The listing builds one solid part. Answer for the finished solid, in the listing's coordinates (mm). Face numbers are marked on the shaded views. A direction names the side the tool comes from. Give positions to 0.01 mm unless a question says otherwise; leave off trailing zeros. Write each loop counter-clockwise with the first axis right and the second up, starting at its lowest first coordinate (ties: lowest second). Pieces come first, ordered by that corner, then holes.
```python
from build123d import *

# Parameters (mm, degrees)
BOSS_EXTRUDE2_DEPTH = 10
FILLET3_R           = 28
SKETCH4_W           = 22
SKETCH4_H           = 48
BOSS_EXTRUDE4_DEPTH = 20
SKETCH9_W           = 18
SKETCH9_H           = 48
BOSS_EXTRUDE6_DEPTH = 60
CUT_EXTRUDE2_DEPTH  = 60
SKETCH12_W          = 18
SKETCH12_H          = 48
BOSS_EXTRUDE7_DEPTH = 60
CUT_EXTRUDE3_START  = -60
CUT_EXTRUDE3_DEPTH  = 60
SKETCH14_R          = 8
CUT_EXTRUDE4_DEPTH  = 140
SKETCH15_R          = 20
CUT_EXTRUDE5_DEPTH  = 140
SKETCH18_R          = 20
BOSS_EXTRUDE9_DEPTH = 12


with BuildPart() as part:
    # Sketch2 → Boss-Extrude2 (new, symmetric)
    with BuildSketch(Plane.XY):
        with BuildLine():
            Line((32, 0), (0, 0))
            Line((0, 0), (0, -56))
            Line((0, -56), (32, -56))
            Line((32, -56), (32, -8))
            Line((32, -8), (89.338383838, -8))
            Line((89.338383838, -8), (108, -8))
            Line((108, -8), (108, -56))
            Line((108, -56), (140, -56))
            Line((140, -56), (140, 0))
            Line((140, 0), (108, 0))
            Line((108, 0), (108, 28))
            ThreePointArc((108, 28), (70, 66), (32, 28))
            Line((32, 28), (32, 0))
        make_face()
    extrude(amount=BOSS_EXTRUDE2_DEPTH, both=True)

    # Fillet3
    fillet3_edges = [part.edges().sort_by_distance(p)[0] for p in [
        (32, 0, 0),
        (108, 0, 0),
    ]]
    fillet(fillet3_edges, radius=FILLET3_R - 0.0001)  # a hair under: the kernel refuses the full size

    # Sketch4 → Boss-Extrude4 (add, through all)
    with BuildSketch(Plane.XY.offset(10)):
        with Locations((97, -32)):
            Rectangle(SKETCH4_W, SKETCH4_H)
        with Locations((43, -32)):
            Rectangle(SKETCH4_W, SKETCH4_H)
    extrude(amount=-BOSS_EXTRUDE4_DEPTH)

    # Sketch9 → Boss-Extrude6 (add)
    with BuildSketch(Plane(origin=(0, 0, -10), x_dir=(-1, 0, 0), z_dir=(0, 0, -1))):
        with Locations((-99, -32)):
            Rectangle(SKETCH9_W, SKETCH9_H)
    extrude(amount=BOSS_EXTRUDE6_DEPTH)

    # Sketch10 → Cut-Extrude2 (cut)
    with BuildSketch(Plane(origin=(108, 0, 0), x_dir=(0, 0, -1), z_dir=(1, 0, 0))):
        with BuildLine():
            Line((70, -8), (10, -8))
            Line((10, -8), (59.189189189, -24.864864865))
            ThreePointArc((59.189189189, -24.864864865), (67.019735539, -30.7001889), (70, -40))
            Line((70, -40), (70, -8))
        make_face()
        with BuildLine():
            Line((70, -56), (70, -40))
            ThreePointArc((70, -40), (65.313708499, -51.313708499), (54, -56))
            Line((54, -56), (70, -56))
        make_face()
    extrude(amount=-CUT_EXTRUDE2_DEPTH, mode=Mode.SUBTRACT)

    # Sketch12 → Boss-Extrude7 (add)
    with BuildSketch(Plane(origin=(0, 0, -10), x_dir=(-1, 0, 0), z_dir=(0, 0, -1))):
        with Locations((-41, -32)):
            Rectangle(SKETCH12_W, SKETCH12_H)
    extrude(amount=BOSS_EXTRUDE7_DEPTH)

    # Sketch13 → Cut-Extrude3 (cut)
    with BuildSketch(Plane.ZY.offset(-32).offset(CUT_EXTRUDE3_START)):
        with BuildLine():
            Line((-70, -8), (-70, -40))
            ThreePointArc((-70, -40), (-67.019735539, -30.7001889), (-59.189189189, -24.864864865))
            Line((-59.189189189, -24.864864865), (-10, -8))
            Line((-10, -8), (-70, -8))
        make_face()
        with BuildLine():
            Line((-70, -40), (-70, -56))
            Line((-70, -56), (-54, -56))
            ThreePointArc((-54, -56), (-65.313708499, -51.313708499), (-70, -40))
        make_face()
    extrude(amount=CUT_EXTRUDE3_DEPTH, mode=Mode.SUBTRACT)

    # Sketch14 → Cut-Extrude4 (cut)
    with BuildSketch(Plane(origin=(108, 0, 0), x_dir=(0, 0, -1), z_dir=(1, 0, 0))):
        with Locations((54, -40)):
            Circle(SKETCH14_R)
    extrude(amount=-CUT_EXTRUDE4_DEPTH, mode=Mode.SUBTRACT)

    # Sketch15 → Cut-Extrude5 (cut)
    with BuildSketch(Plane(origin=(0, 0, -10), x_dir=(-1, 0, 0), z_dir=(0, 0, -1))):
        with Locations((-70, 28)):
            Circle(SKETCH15_R)
    extrude(amount=-CUT_EXTRUDE5_DEPTH, mode=Mode.SUBTRACT)

    # Sketch18 → Boss-Extrude9 (add)
    with BuildSketch(Plane(origin=(0, 0, -10), x_dir=(-1, 0, 0), z_dir=(0, 0, -1))):
        with BuildLine():
            Line((-108, 28), (-108, -8))
            Line((-108, -8), (-32, -8))
            Line((-32, -8), (-32, 28))
            ThreePointArc((-32, 28), (-70, 66), (-108, 28))
        make_face()
        with Locations((-70, 28)):
            Circle(SKETCH18_R, mode=Mode.SUBTRACT)
    extrude(amount=BOSS_EXTRUDE9_DEPTH)


solid = part.part
```
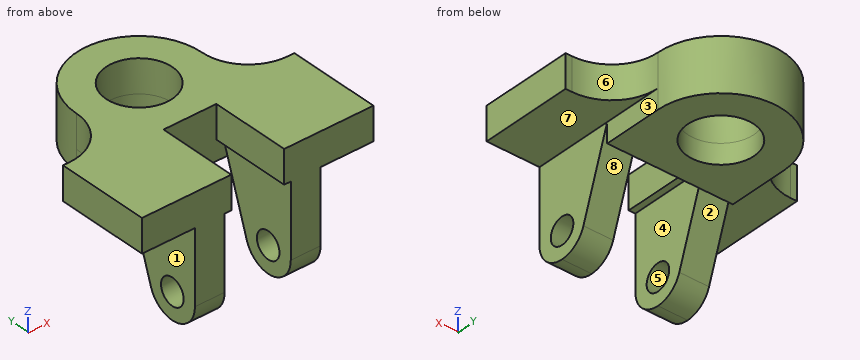
Item 1: A cutting plane is placed at A-A, the plane x = 70. Give the vertices of the cut face in (y, z), plus the area to 3 significant figures.
Conclusion:
outline: (-8, -22) - (8, -22) - (8, 10) - (-8, 10) - close; (48, -22) - (66, -22) - (66, 10) - (48, 10) - close
area: 1,090 mm2
Item 2: A cutting plane is placed at B-B, the plane z = -13. Give the vertices of the cut face in (x, y), plus the area to 3 significant figures.
Conclusion:
outline: (32, -56) - (50, -56) - (50, -9.03) - (32, -9.03) - close; (32, -8) - (108, -8) - (108, 28) arc R38 ccw to (32, 28) - close; (90, -56) - (108, -56) - (108, -9.03) - (90, -9.03) - close; hole circle Ø40 at (70, 28)
area: 5,440 mm2
Item 3: Consider probe 1 along X at (y, z) = (-38, -8); probe 2 along Y at (x, z) = (70, -1.25); probe 3 along X at (y, z) = (-21.5, -36). Determine where each line is inside the solid, lowest interval first.
Conclusion:
probe 1: x = 0 to 54, 86 to 140
probe 2: y = -8 to 8, 48 to 66
probe 3: x = 32 to 50, 90 to 108
Item 4: Each of these flat-tipped pins is pushed along its axis until it touches: P1, Ø2, axis at x = 69.5, z = -22.5, coming from the +Y side; P2, Ø24, axis at y = -20, z = -35, coming from the -X side; P3, Ø16, axis at y = 14.5, z = -6.5, coming from the +X side; P4, Ø24, axis at x = 70, y = 28, coming from the -Z side. Where does it stop, or does it pass through?
Conclusion:
P1: stops at y = 66
P2: stops at x = 32
P3: stops at x = 118.06
P4: passes through
Item 5: A cutting plane is placed at D-D, the plane y = 20. Give the vertices of the cut face in (x, z).
Conclusion:
outline: (30.83, -10) - (32, -10) - (32, -22) - (51.67, -22) - (51.67, 10) - (30.83, 10) - close; (88.33, -22) - (108, -22) - (108, -10) - (109.17, -10) - (109.17, 10) - (88.33, 10) - close
Item 6: Which of the six approach directions +Z, -Z, +X, -X, +Y, -Y give full straight-line access (tool end or side, diameter ignored) to the marked faces 1, 2, 3 and 4?
Conclusion:
face 1: -Z, -X, +Y, -Y
face 2: -Z, +X, -X
face 3: -Z, +X, +Y, -Y
face 4: -Z, -Y
Item 7: Determine the mould class of the marked faces 5, 6, 7 and 8 for opening direction Y: pulls with the +Y half, pulls with the -Y half, needs draft (parallel to the pull), parting line crosses it, or undercut.
Conclusion:
face 5: undercut
face 6: pulls with the +Y half
face 7: needs draft
face 8: undercut
